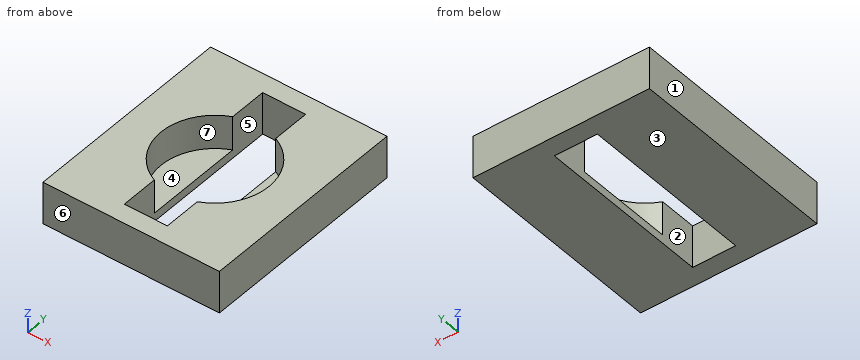
```python
from build123d import *

# Parameters (mm, degrees)
F0_W     = 50
F0_H     = 60
F1_DEPTH = 12
F2_DEPTH = 2.4


with BuildPart() as f1:
    # F0 (on Top) → F1 (new body)
    with BuildSketch(Plane.XY):
        Rectangle(F0_W, F0_H)
        with BuildLine():
            Line((6.1, -14.0313933734), (6.1, -24.75))
            Line((6.1, -24.75), (-6.1, -24.75))
            Line((-6.1, -24.75), (-6.1, -14.0313933734))
            ThreePointArc((-6.1, -14.0313933734), (-15.3, 0), (-6.1, 14.0313933734))
            Line((-6.1, 14.0313933734), (-6.1, 24.75))
            Line((-6.1, 24.75), (6.1, 24.75))
            Line((6.1, 24.75), (6.1, 14.0313933734))
            ThreePointArc((6.1, 14.0313933734), (12.7949208673, 8.3892788725), (15.3, 0))
            ThreePointArc((15.3, 0), (12.7949208673, -8.3892788725), (6.1, -14.0313933734))
        make_face(mode=Mode.SUBTRACT)
    extrude(amount=F1_DEPTH)

    # F0 (on Top) → F2 (join)
    with BuildSketch(Plane.XY):
        with BuildLine():
            ThreePointArc((-6.1, 14.0313933734), (-15.3, 0), (-6.1, -14.0313933734))
            Line((-6.1, -14.0313933734), (-6.1, 14.0313933734))
        make_face()
        with BuildLine():
            Line((6.1, 14.0313933734), (6.1, -14.0313933734))
            ThreePointArc((6.1, -14.0313933734), (12.7949208673, -8.3892788725), (15.3, 0))
            ThreePointArc((15.3, 0), (12.7949208673, 8.3892788725), (6.1, 14.0313933734))
        make_face()
    extrude(amount=F2_DEPTH)


solid = f1.part
```
Here's how the part is built. I have some questions about the finished solid (model axes, mm). Face numbers are marked on the shaded views. A direction names the side the tool comes from. Round coordinates to 2 decimals unless told otherwise and drop trailing zeros. Loops run counter-clockwise (first coordinate to the right, second up) from the corner with the lowest first, then second, coordinate; pieces in that order, holes last. Notation, with made-up numbers: (54.5, 66.25) -> (98.5, 66.25) arc R6 ccw to (98.5, 72.25) -> close; hole circle Ø7 at (48, 46.25). An arc over 180 degrees is marked (long way). Answer as CSV lines item,"result".
1. If we section it at C-C on z = 8.75: Please give me the cut outline in (x, y), plus the area to 3 significant figures.
Final values:
outline,"(-25, -30) -> (25, -30) -> (25, 30) -> (-25, 30) -> close; hole (-6.1, -24.75) -> (6.1, -24.75) -> (6.1, -14.03) arc R15.3 ccw to (6.1, 14.03) -> (6.1, 24.75) -> (-6.1, 24.75) -> (-6.1, 14.03) arc R15.3 ccw to (-6.1, -14.03) -> close"
area,"2,020 mm^2"
2. For pin 1 (7.5 mm diameter, centred on x = -9, y = 4, fed in from +Z); pin 2 (2 mm diameter, centred on x = -4, y = -7.5, fed in from -Z); pin 3 (12 mm diameter, centred on x = 6, y = -9, fed in from +Z), each with a flat end and sliding along its axis, tell me the tip position at first contact or that it passes through.
Final values:
pin 1,"stops at z = 2.4"
pin 2,"passes through"
pin 3,"stops at z = 12"
3. If we section it at A-A on y = -22: Please give me the cut outline in (x, z), plus the area to 3 significant figures.
Final values:
outline,"(-25, 0) -> (-6.1, 0) -> (-6.1, 12) -> (-25, 12) -> close; (6.1, 0) -> (25, 0) -> (25, 12) -> (6.1, 12) -> close"
area,"454 mm^2"
4. If we section it at B-B on x = 4.5: Please give me the cut outline in (y, z).
Final values:
outline,"(-30, 0) -> (-24.75, 0) -> (-24.75, 12) -> (-30, 12) -> close; (24.75, 0) -> (30, 0) -> (30, 12) -> (24.75, 12) -> close"
5. If I drill on L1, parallel to Y at x = 1, z = 2.5; L2, parallel to X at y = 19, z = 1.5; L3, parallel to X at y = 0, z = 6, over which ranges is the centre line in solid material (lowest first)?
Final values:
L1,"y = -30 to -24.75, 24.75 to 30"
L2,"x = -25 to -6.1, 6.1 to 25"
L3,"x = -25 to -15.3, 15.3 to 25"
6. If we section it at D-D on y = 3.5: Please give me the cut outline in (x, z).
Final values:
outline,"(-25, 0) -> (-6.1, 0) -> (-6.1, 2.4) -> (-14.89, 2.4) -> (-14.89, 12) -> (-25, 12) -> close; (6.1, 0) -> (25, 0) -> (25, 12) -> (14.89, 12) -> (14.89, 2.4) -> (6.1, 2.4) -> close"
7. Which directions (+Z, -Z, +X, -X, +Y, -Y) give clear straight access to the entire face, cutting with the end or side of a thin tool? Please do the marked faces 5, 6 and 7.
Final values:
face 5,"+Z, -Z"
face 6,"+Z, -Z, +X, -X, -Y"
face 7,"+Z"
8. Thinking about a two-plate mould opening in X: for the marked faces 1, 2, 3 and 4, which applies, released by +X, released by -X, zero draft, split by the parting line, or undercut?
Final values:
face 1,"released by -X"
face 2,"undercut"
face 3,"zero draft"
face 4,"undercut"
